```python
from build123d import *

# Parameters (mm, degrees)
BOSS_EXTRUDE1_DEPTH = 6.35
SHELL1_T            = -2.032


with BuildPart() as part:
    # Sketch1 → Boss-Extrude1 (new body)
    with BuildSketch(Plane(origin=(0, 0, 0), x_dir=(1, 0, 0), z_dir=(0, 1, 0))):
        with BuildLine():
            Line((0, -113.792), (0, 0))
            ThreePointArc((0, 0), (-25.836593541, -56.896), (0, -113.792))
        make_face()
    extrude(amount=BOSS_EXTRUDE1_DEPTH)

    # Shell1
    shell1_openings = [part.faces().sort_by_distance(p)[0] for p in [
        (-12.91829677, 6.35, 56.896),
    ]]
    offset(amount=SHELL1_T, openings=shell1_openings)


solid = part.part
```
The listing builds one solid part. Answer for the finished solid, in the listing's coordinates (mm). A direction names the side the tool comes from. Give positions to 0.01 mm unless a question says otherwise; leave off trailing zeros. Loops run counter-clockwise (first coordinate to the right, second up) from the corner with the lowest first, then second, coordinate; pieces in that order, holes last. Notation, with made-up numbers: M -22,-30.5 L 20,-30.5 A5 cw 20,-25.5 Z; hole C 71.25,-38.75 d7. An arc over 180 degrees is marked long. One line per item, written item: value.
Q1. A cutting plane is placed at A-A on y = 4. Determine the outline of the cut face in (x, z) (3 decimals), then the cut area to 3 significant figures.
Working result:
outline: M 0,0 L 0,113.792 A75.565 ccw Z; hole M -2.032,4.666 L -2.032,109.126 A73.533 ccw Z
area: 471 mm^2
Q2. A cutting plane is placed at B-B on x = -22. Determine the outline of the cut face in (y, z).
Working result:
outline: M 0,33.12 L 6.35,33.12 L 6.35,40.71 L 2.03,40.71 L 2.03,73.09 L 6.35,73.09 L 6.35,80.67 L 0,80.67 Z
Q3. For faces 4 (the face through (-1, 6.35, 57)), 5 (the face through (-2.032, 4, 58)), determine the directions among +Z, -Z, +X, -X, +Y, -Y from which every point of the face is accessible in a straight line to the end or side of a thin tool.
Working result:
face 4: +Z, -Z, +X, -X, +Y
face 5: +Y
Q4. A cutting plane is placed at C-C on z = 92.5. Determine the outline of the cut face in (x, y), then the cut area to 3 significant figures.
Working result:
outline: M -16.92,0 L 0,0 L 0,6.35 L -2.03,6.35 L -2.03,2.03 L -14.61,2.03 L -14.61,6.35 L -16.92,6.35 Z
area: 53.1 mm^2
Q5. Find the intervals of material crossed by line 1 (X direction, y = 5, z = 58.5); line 2 (X direction, y = 5.25, z = 29); line 3 (Y direction, x = -17, z = 61), in increasing order. Write a range as from..to.
Working result:
line 1: x = -25.82..-23.79, -2.03..0
line 2: x = -20.5..-18.31, -2.03..0
line 3: y = 0..2.03
Q6. Flat-ended cylindrical pins translate along their axes: P1, Ø3, axis at x = -7.5, z = 41.5, coming from the +Y side; P2, Ø2, axis at x = -11.5, y = 0.5, coming from the +Z side; P3, Ø2, axis at y = 4, z = 51.5, coming from the -X side. Find the tip coordinate at first contact, or state that the pin passes through.
Working result:
P1: stops at y = 2.03
P2: stops at z = 102.53
P3: stops at x = -25.71
Q7. Determine the mould class of faces 1 (the face through (-10, 0, 56)), 2 (the face through (-25.83, 3.13, 55.99)), 3 (the face through (-23.8, 4.2, 56.1)) for opening direction X: +X half, -X half, draft (parallel to the pull), parting line (faces both ways), or undercut.
Working result:
face 1: draft
face 2: -X half
face 3: undercut
